```python
from build123d import *

# Parameters (mm, degrees)
PAD_DEPTH       = 2
PAD001_DEPTH    = 5.4
PAD002_DEPTH    = 7.9
SKETCH003_W     = 10
SKETCH003_H     = 2
POCKET_DEPTH    = 1.8
SKETCH004_W     = 2
SKETCH004_H     = 15
PAD003_DEPTH    = 1.5
SKETCH005_W     = 5
SKETCH005_H     = 1.5
POCKET001_DEPTH = 1.2
SKETCH006_W     = 5
SKETCH006_H     = 1.5
POCKET002_DEPTH = 1.2
SKETCH007_W     = 5
SKETCH007_H     = 1.5
POCKET003_DEPTH = 1.2


with BuildPart() as part:
    # Sketch → Pad (new body)
    with BuildSketch(Plane.XY):
        with BuildLine():
            Line((149.259997, 103.29), (149.259997, 4))
            ThreePointArc((145.259999, 0), (148.088425, 1.171573), (149.259997, 4))
            Line((3.999999, 0), (145.259999, 0))
            ThreePointArc((0, 4), (1.171572, 1.171573), (3.999999, 0))
            Line((0, 103.29), (0, 4))
            ThreePointArc((3.999997, 107.29), (1.171572, 106.118426), (0, 103.29))
            Line((3.999997, 107.29), (145.259997, 107.29))
            ThreePointArc((149.259997, 103.29), (148.088425, 106.118427), (145.259997, 107.29))
        make_face()
    extrude(amount=PAD_DEPTH)

    # Sketch001 (on Face10 of Pad) → Pad001 (join)
    with BuildSketch(Plane.XY.offset(2)):
        with BuildLine():
            ThreePointArc((149.259997, 103.29), (148.088425, 106.118427), (145.259997, 107.29))
            Line((3.999998, 107.29), (145.259997, 107.29))
            ThreePointArc((3.999998, 107.29), (1.171572, 106.118426), (0, 103.29))
            Line((0, 3.999998), (0, 103.29))
            ThreePointArc((0, 3.999998), (1.171573, 1.171573), (3.999999, 0))
            Line((145.259996, 0), (3.999999, 0))
            ThreePointArc((145.259996, 0), (148.088424, 1.171572), (149.259997, 4))
            Line((149.259997, 103.29), (149.259997, 4))
        make_face()
        with BuildLine():
            Line((3.999998, 105.49), (145.259995, 105.49))
            ThreePointArc((147.459997, 103.290002), (146.815631, 104.845636), (145.259995, 105.49))
            Line((147.459997, 4.000002), (147.459997, 103.290002))
            ThreePointArc((145.26, 1.8), (146.815634, 2.444367), (147.459997, 4.000002))
            Line((4.000003, 1.8), (145.26, 1.8))
            ThreePointArc((1.8, 3.999996), (2.444368, 2.444363), (4.000003, 1.8))
            Line((1.8, 103.289998), (1.8, 3.999996))
            ThreePointArc((3.999998, 105.49), (2.444364, 104.845634), (1.8, 103.289998))
        make_face(mode=Mode.SUBTRACT)
    extrude(amount=PAD001_DEPTH)

    # Sketch002 (on Face10 of Pad001) → Pad002 (join)
    with BuildSketch(Plane.XY.offset(2)):
        with BuildLine():
            Line((145.709997, 103.74), (145.709997, 3.55))
            Line((145.709997, 3.55), (3.55, 3.55))
            Line((3.55, 3.55), (3.55, 63.55))
            Line((3.55, 63.55), (1.8, 63.55))
            Line((1.8, 63.55), (1.8, 3.999996))
            ThreePointArc((1.8, 3.999996), (2.444368, 2.444363), (4.000003, 1.8))
            Line((4.000003, 1.8), (145.26, 1.8))
            ThreePointArc((145.26, 1.8), (146.815634, 2.444367), (147.459997, 4.000003))
            Line((147.459997, 4.000003), (147.459997, 103.290002))
            ThreePointArc((147.459997, 103.290002), (146.815631, 104.845636), (145.259995, 105.49))
            Line((145.259995, 105.49), (27.8, 105.49))
            Line((27.8, 105.49), (27.8, 103.74))
            Line((27.8, 103.74), (145.709997, 103.74))
        make_face()
    extrude(amount=PAD002_DEPTH)

    # Sketch003 (on Face5 of Pad002) → Pocket (cut)
    with BuildSketch(Plane(origin=(0, 0, 0), x_dir=(0, -1, 0), z_dir=(-1, 0, 0))):
        with Locations((-78.29, 6.4)):
            Rectangle(SKETCH003_W, SKETCH003_H)
    extrude(amount=-POCKET_DEPTH, mode=Mode.SUBTRACT)

    # Sketch004 (on Face24 of Pocket) → Pad003 (join)
    with BuildSketch(Plane.XY.offset(2)):
        with Locations((4.8, 78.29)):
            Rectangle(SKETCH004_W, SKETCH004_H)
    extrude(amount=PAD003_DEPTH)

    # Sketch005 (on Face13 of Pad003) → Pocket001 (cut)
    with BuildSketch(Plane.YZ.offset(147.459997)):
        with Locations((11.3, 8.15)):
            Rectangle(SKETCH005_W, SKETCH005_H)
        with Locations((95.99, 8.15)):
            Rectangle(SKETCH005_W, SKETCH005_H)
    extrude(amount=-POCKET001_DEPTH, mode=Mode.SUBTRACT)

    # Sketch006 (on Face18 of Pocket001) → Pocket002 (cut)
    with BuildSketch(Plane(origin=(1.8, 0, 0), x_dir=(0, -1, 0), z_dir=(-1, 0, 0))):
        with Locations((-54.05, 8.15)):
            Rectangle(SKETCH006_W, SKETCH006_H)
        with Locations((-11.3, 8.15)):
            Rectangle(SKETCH006_W, SKETCH006_H)
    extrude(amount=-POCKET002_DEPTH, mode=Mode.SUBTRACT)

    # Sketch007 (on Face21 of Pocket002) → Pocket003 (cut)
    with BuildSketch(Plane(origin=(0, 105.49, 0), x_dir=(-1, 0, 0), z_dir=(0, 1, 0))):
        with Locations((-37.3, 8.15)):
            Rectangle(SKETCH007_W, SKETCH007_H)
    extrude(amount=-POCKET003_DEPTH, mode=Mode.SUBTRACT)


solid = part.part
```
Model file for the job. Use its own axes, mm. A direction names the side the tool comes from. Coordinates: 2 decimals unless noted, no trailing zeros. Write each loop counter-clockwise with the first axis right and the second up, starting at its lowest first coordinate (ties: lowest second). Pieces come first, ordered by that corner, then holes. Notation, with made-up numbers: (76, 40.5) - (112, 40.5) arc R10 cw to (112, 44.5) - close; hole circle Ø10 at (13.25, 17). An arc over 180 degrees is marked (long way). One line per item, written item: value. Start each with the question number.
1. Tool access for faces 1 (the flat face through (74, 107.29, 4)), 2 (the flat face through (1.8, 84, 5)): list every direction of +Z, -Z, +X, -X, +Y, -Y with a clear straight run to the whole face (end or side of a thin tool).
2. Probe line 1 (X direction, y = 78.5, z = 2.75); line 2 (Y direction, x = 42, z = 3.75); line 3 (X direction, y = 26, z = 3.5). List the from-to ranges inside material, lowest first. Write a range as from..to.
3. Slice it at A-A (x = 54). Write the cut outline in (y, z).
4. Slice it at C-C (x = 14). Write the cut outline in (y, z).
5. Flat gauge pins, fed straight in: pin 1 (0.6 mm diameter, centred on x = 147, z = 8, fed in from +Y); pin 2 (1.6 mm diameter, centred on x = 4.5, y = 80.5, fed in from +Z); pin 3 (2 mm diameter, centred on x = 1, y = 80, fed in from +Z). Where does each tip first touch, or does it go through?
6. Slice it at D-D (y = 42). Write the cut outline in (x, z).
7. Slice it at B-B (y = 75). Write the cut outline in (x, z).
8. Mould opens along X. For faces 3 (the flat face through (90, 104, 9.9)), 4 (the cylindrical face through (148.119, 106.087, 3.648)), 5 (the flat face through (145.71, 54, 6)) say: released by +X, released by -X, zero draft, split by the parting line, or undercut.
Answers below:
1. face 1: +Z, -Z, +X, -X, +Y
1. face 2: +Z
2. line 1: x = 0..1.8, 3.8..5.8, 145.71..149.26
2. line 2: y = 0..3.55, 103.74..107.29
2. line 3: x = 0..3.55, 145.71..149.26
3. outline: (0, 0) - (107.29, 0) - (107.29, 7.4) - (105.49, 7.4) - (105.49, 9.9) - (103.74, 9.9) - (103.74, 2) - (3.55, 2) - (3.55, 9.9) - (1.8, 9.9) - (1.8, 7.4) - (0, 7.4) - close
4. outline: (0, 0) - (107.29, 0) - (107.29, 7.4) - (105.49, 7.4) - (105.49, 2) - (3.55, 2) - (3.55, 9.9) - (1.8, 9.9) - (1.8, 7.4) - (0, 7.4) - close
5. pin 1: stops at y = 104.95
5. pin 2: stops at z = 3.5
5. pin 3: stops at z = 5.4
6. outline: (0, 0) - (149.26, 0) - (149.26, 7.4) - (147.46, 7.4) - (147.46, 9.9) - (145.71, 9.9) - (145.71, 2) - (3.55, 2) - (3.55, 9.9) - (1.8, 9.9) - (1.8, 7.4) - (0, 7.4) - close
7. outline: (0, 0) - (149.26, 0) - (149.26, 7.4) - (147.46, 7.4) - (147.46, 9.9) - (145.71, 9.9) - (145.71, 2) - (5.8, 2) - (5.8, 3.5) - (3.8, 3.5) - (3.8, 2) - (1.8, 2) - (1.8, 5.4) - (0, 5.4) - close
8. face 3: zero draft
8. face 4: released by +X
8. face 5: undercut
